Read the model definition and answer for the solid it produces. Units are mm, in the model's axes. A direction names the side the tool comes from. Coordinates: 2 decimals unless noted, no trailing zeros. Write each loop counter-clockwise with the first axis right and the second up, starting at its lowest first coordinate (ties: lowest second). Pieces come first, ordered by that corner, then holes. Notation, with made-up numbers: (-7, 79.25) - (47, 79.25) arc R26 ccw to (47, 95.25) - close; hole circle Ø9 at (-24.75, 15.5). An arc over 180 degrees is marked (long way). Return JSON: item names as keys, results as strings.
Autodesk Inventor part; units mm, degrees
ref_plane "YZ Plane" through (0, 0, 0) normal (1, 0, 0) x (0, 1, 0)
ref_plane "XZ Plane" through (0, 0, 0) normal (0, 1, 0) x (-1, 0, 0)
ref_plane "XY Plane" through (0, 0, 0) normal (0, 0, 1) x (1, 0, 0)
sketch "Sketch1" plane through (0, 0, 0) normal (0, 0, 1) x (1, 0, 0)
  line L0 (-117.5, 54) -> (117.5, 54)
  line L1 (117.5, 54) -> (117.5, -54)
  line L2 (117.5, -54) -> (-117.5, -54)
  line L3 (-117.5, -54) -> (-117.5, 54)
  line L4 (-88.19, 36) -> (117.5, 36)
  line L5 (117.5, 36) -> (117.5, -36)
  line L6 (117.5, -36) -> (-88.19, -36)
  line L7 (-88.19, -36) -> (-88.19, 36)
  point P0 (0, 0)
  point P1 (117.5, 0)
  point P2 (0, 54)
  point P3 (117.5, 0)
  point P4 (117.5, -36)
  dimension "d0" = 108
  dimension "d1" = 235
  dimension "d4" = 205.69
  dimension "d5" = 72
extrude "Extrusion2" add sketch "Sketch1" against normal blind 10 contours L1 L6 L7 L4
extrude "Extrusion3" add sketch "Sketch1" along normal blind 10
chamfer "Chamfer1" distance 2 angle 45 4 edges at (14.655, -36, -10) (14.655, 36, -10) (-88.19, 0, -10) (117.5, 0, -10)
fillet "Fillet1" radius 5 2 edges at (0, 54, 10) (0, -54, 10)
sketch "Sketch3" plane through (0, 0, 10) normal (0, 0, 1) x (1, 0, 0)
  line L0 (117.5, -49) -> (-117.5, -49)
  line L1 (-117.5, 49) -> (117.5, 49)
  line L2 (-117.5, -54) -> (117.5, -54)
  line L3 (117.5, 54) -> (-117.5, 54)
  line L4 (-117.5, 49) -> (-117.5, -49)
  line L5 (117.5, -49) -> (117.5, 49)
  point P0 (-103.7107, 43.9255)
  point P1 (-103.7107, 0)
  point P2 (-103.7107, -43.9255)
  point P3 (-117.5, 0)
  dimension "d18" = 98
  dimension "d19" = 108
  dimension "d20" = 87.851
  dimension "d21" = 43.9255
  dimension "d22" = 221.2107
hole "Hole1" at (-103.7107, 43.9255, 10) at (-103.7107, -43.9255, 10) direction (0, 0, -1) diameter 18 depth 50 tip angle 118
pattern_linear "Rectangular Pattern1" count 5 spacing 50 along (1, 0, 0) of "Hole1"
hole "Hole2" at (-103.7107, 0, 10) direction (0, 0, -1) diameter 18 depth 15 tip angle 118
properties part number "Cover part of robot arm bottom side" material "Steel, Alloy"
(1) A cutting plane is placed at C-C (y = -20). Determine the outline of the cut face in (x, z).
Answer:
{"outline": "(-117.5, 0) - (-88.19, 0) - (-88.19, -8) - (-86.19, -10) - (115.5, -10) - (117.5, -8) - (117.5, 10) - (-117.5, 10) - close"}
(2) Straight lines are drawn through the part: line 1 (X direction, y = 43, z = 4.5); line 2 (X direction, y = -44, z = 6.25); line 3 (X direction, y = 0, z = 8.25). For each, find the intervals that lie inside material, in ascending order. Write a range as from..to.
Answer:
{"line 1": "-117.5..-112.66, -94.76..-62.66, -44.76..-12.66, 5.24..37.34, 55.24..87.34, 105.24..117.5", "line 2": "-117.5..-112.71, -94.71..-62.71, -44.71..-12.71, 5.29..37.29, 55.29..87.29, 105.29..117.5", "line 3": "-117.5..-112.71, -94.71..117.5"}
(3) A cutting plane is placed at A-A (y = 0). Determine the outline of the cut face in (x, z).
Answer:
{"outline": "(-117.5, 0) - (-112.71, 0) - (-112.71, 10) - (-117.5, 10) - close; (-94.71, 0) - (-88.19, 0) - (-88.19, -8) - (-86.19, -10) - (115.5, -10) - (117.5, -8) - (117.5, 10) - (-94.71, 10) - close"}
(4) Determine the mould class of faces 4 (the face through (-50.264, 35.612, 2.449)), 5 (the face through (109, 36, -4)), 6 (the face through (-26.7, 36.3, 0)) for opening direction Y: +Y half, -Y half, draft (parallel to the pull), parting line (faces both ways), or undercut.
Answer:
{"face 4": "undercut", "face 5": "+Y half", "face 6": "draft"}
(5) Flat-ended cylindrical pins translate along their axes: P1, Ø4, axis at x = 76.5, z = -3.5, coming from the +Y side; P2, Ø2, axis at y = 37.5, z = -2, coming from the -X side; P3, Ø6.5, axis at x = 110, z = -4, coming from the -Y side; P4, Ø20.5, axis at x = -103.71, y = -43.93, coming from the -Z side. Find the tip coordinate at first contact, or state that the pin passes through.
Answer:
{"P1": "y = 36", "P2": "through", "P3": "y = -36", "P4": "z = 0"}
(6) Which of the six approach directions +Z, -Z, +X, -X, +Y, -Y give full straight-line access (tool end or side, diameter ignored) to faces 1 (the face through (-73, -36, -4)), 2 (the face through (-73, 36, -4)), 3 (the face through (-88.19, -1, -4))?
Answer:
{"face 1": "-Z, +X, -X, -Y", "face 2": "-Z, +X, -X, +Y", "face 3": "-Z, -X, +Y, -Y"}
(7) A cutting plane is placed at B-B (x = 12.5). Determine the outline of the cut face in (y, z).
Answer:
{"outline": "(-54, 0) - (-36, 0) - (-36, -8) - (-34, -10) - (34, -10) - (36, -8) - (36, 0) - (54, 0) - (54, 5) arc R5 ccw to (49, 10) - (-49, 10) arc R5 ccw to (-54, 5) - close"}
